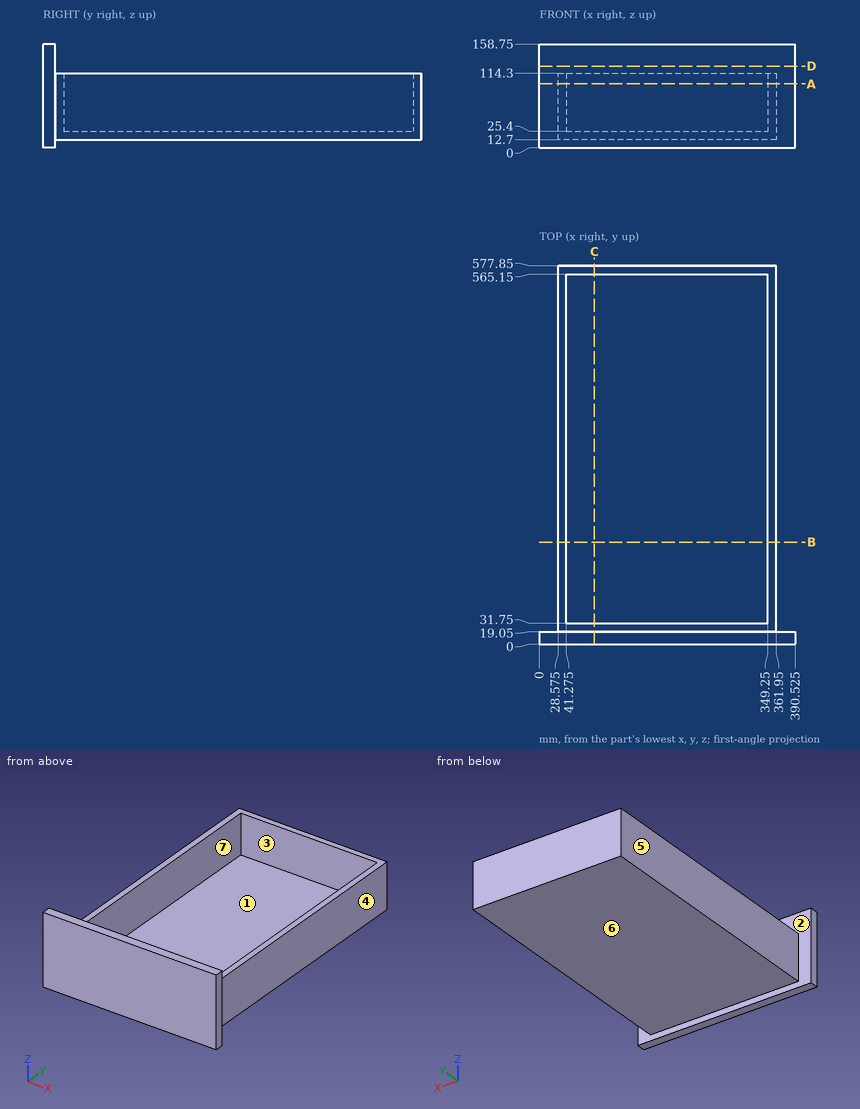
For this review, use the dimensioned drawing (mm, ordinates from the lowest corner) and the shaded views. A direction names the side the tool comes from. Give positions to 0.01 mm unless a question says otherwise; leave off trailing zeros. Loops run counter-clockwise (first coordinate to the right, second up) from the corner with the lowest first, then second, coordinate; pieces in that order, holes last. Notation, with made-up numbers: (64, 38.5) - (71, 38.5) arc R30 ccw to (71, 66.5) - close; hole circle Ø10 at (73, 30.25). An arc over 180 degrees is marked (long way). Write each question's results on one line, items separated by ' | '.
(1) For line 1 along X through (y, z) = (80.5, 73.5) (3 decimals); line 2 along Y through (x, z) = (96, 78); line 3 along Z through (x, y) = (185.5, 137), list the stretches that pass through material, from the lowest coordinate up.
Conclusion:
line 1: 28.575 to 41.275, 349.25 to 361.95 | line 2: 0 to 31.75, 565.15 to 577.85 | line 3: 12.7 to 25.4
(2) Take a section at D-D (z = 125). Give the boundary of the cut face in (x, y) (3 decimals), then the cut area to 3 significant figures.
Conclusion:
outline: (0, 0) - (390.525, 0) - (390.525, 19.05) - (0, 19.05) - close | area: 7,440 mm^2
(3) For the marked faces 5, 6 and 7, list the 3-axis set-ups (+Z, -Z, +X, -X, +Y, -Y) from which the entire face can be reached by the end or side of a thin tool; tool diameter is ignored.
Conclusion:
face 5: +Z, -Z, -X, +Y | face 6: -Z, +X, -X, +Y | face 7: +Z
(4) Take a section at A-A (z = 98). Give the boundary of the cut face in (x, y) (3 decimals), then the cut area to 3 significant figures.
Conclusion:
outline: (0, 0) - (390.525, 0) - (390.525, 19.05) - (361.95, 19.05) - (361.95, 577.85) - (28.575, 577.85) - (28.575, 19.05) - (0, 19.05) - close; hole (41.275, 31.75) - (349.25, 31.75) - (349.25, 565.15) - (41.275, 565.15) - close | area: 29,500 mm^2
(5) Take a section at B-B (y = 156). Give the boundary of the cut face in (x, z) (3 decimals).
Conclusion:
outline: (28.575, 12.7) - (361.95, 12.7) - (361.95, 114.3) - (349.25, 114.3) - (349.25, 25.4) - (41.275, 25.4) - (41.275, 114.3) - (28.575, 114.3) - close
(6) Take a section at C-C (x = 84). Give the boundary of the cut face in (y, z).
Conclusion:
outline: (0, 0) - (19.05, 0) - (19.05, 12.7) - (577.85, 12.7) - (577.85, 114.3) - (565.15, 114.3) - (565.15, 25.4) - (31.75, 25.4) - (31.75, 114.3) - (19.05, 114.3) - (19.05, 158.75) - (0, 158.75) - close
(7) Draft analysis for pull direction X (two halves, no side actions). For the marked faces 1, 2, 3 and 4, state which applies: +X half, -X half, draft (parallel to the pull), parting line (faces both ways), or undercut.
Conclusion:
face 1: undercut | face 2: draft | face 3: undercut | face 4: +X half
(8) For pin 1 Ø12 at (x, z) = (46, 86) entering from -Y; pin 2 Ø8 at (y, z) = (142, 67) entering from +X; pin 3 Ø5 at (x, y) = (124, 393.5) entering from +Z; pin 4 Ø4 at (y, z) = (206, 112) entering from -X (3 decimals), all flat-tipped, find the tip position at first contact; note any pin that passes through.
Conclusion:
pin 1: y = 0 | pin 2: x = 361.95 | pin 3: z = 25.4 | pin 4: x = 28.575
